CAD build for the part. Positions are in the model's coordinates, mm. A direction names the side the tool comes from. Give positions to 0.01 mm unless a question says otherwise; leave off trailing zeros. Write each loop counter-clockwise with the first axis right and the second up, starting at its lowest first coordinate (ties: lowest second). Pieces come first, ordered by that corner, then holes. Notation, with made-up numbers: (21, -4) -> (28, -4) arc R18 cw to (28, 27) -> close; hole circle Ø11 at (24.25, -34.5). An arc over 180 degrees is marked (long way). Answer in a Markdown table with one row per item. Add a question column.
```python
from build123d import *

# Parameters (mm, degrees)
SKETCH1_W           = 115
SKETCH1_H           = 70
BOSS_EXTRUDE1_DEPTH = 10
SKETCH2_R           = 6.3
SKETCH2_R_2         = 1.5
CUT_EXTRUDE1_DEPTH  = 10
SKETCH3_R           = 18.5
CUT_EXTRUDE2_DEPTH  = 5
SKETCH4_R           = 2
CUT_EXTRUDE3_DEPTH  = 10
CUT_EXTRUDE4_START  = -10
SKETCH5_R           = 2
CUT_EXTRUDE4_DEPTH  = 10
SKETCH6_R           = 2
CUT_EXTRUDE5_DEPTH  = 5
SKETCH7_R           = 2
CUT_EXTRUDE6_DEPTH  = 10


with BuildPart() as part:
    # Sketch1 → Boss-Extrude1 (new body)
    with BuildSketch(Plane(origin=(0, 0, 0), x_dir=(1, 0, 0), z_dir=(0, 1, 0))):
        Rectangle(SKETCH1_W, SKETCH1_H)
    extrude(amount=BOSS_EXTRUDE1_DEPTH)

    # Sketch2 → Cut-Extrude1 (cut)
    with BuildSketch(Plane(origin=(0, 10, 0), x_dir=(1, 0, 0), z_dir=(0, 1, 0))):
        with Locations(Location((0, -22.5, 0), (0, 0, 270))):
            Circle(SKETCH2_R)
        with Locations(Location((15.5, -15.5, 0), (0, 0, 270))):
            Circle(SKETCH2_R_2)
        with Locations(Location((7.75, -28.923393759, 0), (0, 0, 270))):
            Circle(SKETCH2_R_2)
        with Locations(Location((-7.75, -28.923393759, 0), (0, 0, 270))):
            Circle(SKETCH2_R_2)
        with Locations(Location((-15.5, -15.5, 0), (0, 0, 270))):
            Circle(SKETCH2_R_2)
        with Locations(Location((-7.75, -2.076606241, 0), (0, 0, 270))):
            Circle(SKETCH2_R_2)
        with Locations(Location((7.75, -2.076606241, 0), (0, 0, 270))):
            Circle(SKETCH2_R_2)
    extrude(amount=-CUT_EXTRUDE1_DEPTH, mode=Mode.SUBTRACT)

    # Sketch3 → Cut-Extrude2 (cut)
    with BuildSketch(Plane.XZ):
        with Locations(Location((0, 15.5, 0), (0, 0, 270))):
            Circle(SKETCH3_R)
    extrude(amount=-CUT_EXTRUDE2_DEPTH, mode=Mode.SUBTRACT)

    # Sketch4 → Cut-Extrude3 (cut)
    with BuildSketch(Plane.ZY.offset(57.5)):
        with Locations((30, 5)):
            Circle(SKETCH4_R)
        with Locations((15, 5)):
            Circle(SKETCH4_R)
        with Locations((-5, 5)):
            Circle(SKETCH4_R)
        with Locations((-25, 5)):
            Circle(SKETCH4_R)
    extrude(amount=-CUT_EXTRUDE3_DEPTH, mode=Mode.SUBTRACT)

    # Sketch5 → Cut-Extrude4 (cut)
    with BuildSketch(Plane(origin=(57.5, 0, 0), x_dir=(0, 0, -1), z_dir=(1, 0, 0)).offset(CUT_EXTRUDE4_START)):
        with Locations(Location((-30, 5, 0), (0, 0, 180))):
            Circle(SKETCH5_R)
        with Locations(Location((-15, 5, 0), (0, 0, 180))):
            Circle(SKETCH5_R)
        with Locations(Location((5, 5, 0), (0, 0, 180))):
            Circle(SKETCH5_R)
        with Locations(Location((25, 5, 0), (0, 0, 180))):
            Circle(SKETCH5_R)
    extrude(amount=CUT_EXTRUDE4_DEPTH, mode=Mode.SUBTRACT)

    # Sketch6 → Cut-Extrude5 (cut)
    with BuildSketch(Plane(origin=(0, 0, -35), x_dir=(-1, 0, 0), z_dir=(0, 0, -1))):
        with Locations((-52.5, 5)):
            Circle(SKETCH6_R)
        with Locations((52.5, 5)):
            Circle(SKETCH6_R)
    extrude(amount=-CUT_EXTRUDE5_DEPTH, mode=Mode.SUBTRACT)

    # Sketch7 → Cut-Extrude6 (cut)
    with BuildSketch(Plane.XZ):
        with Locations(Location((42.5, 20, 0), (0, 0, 270))):
            Circle(SKETCH7_R)
        with Locations(Location((42.5, 0, 0), (0, 0, 270))):
            Circle(SKETCH7_R)
        with Locations(Location((42.5, -20, 0), (0, 0, 270))):
            Circle(SKETCH7_R)
        with Locations(Location((-42.5, -20, 0), (0, 0, 270))):
            Circle(SKETCH7_R)
        with Locations(Location((-42.5, 0, 0), (0, 0, 270))):
            Circle(SKETCH7_R)
        with Locations(Location((-42.5, 20, 0), (0, 0, 270))):
            Circle(SKETCH7_R)
        with Locations(Location((0, -20, 0), (0, 0, 270))):
            Circle(SKETCH7_R)
    extrude(amount=-CUT_EXTRUDE6_DEPTH, mode=Mode.SUBTRACT)


solid = part.part
```
Item 1: Mould opens along Z. For faces 6 (the face through (-44.452, 4.93, 20.434)), 7 (the face through (-1, 5, -35)), 8 (the face through (57.5, 5, 0)) say: released by +Z, released by -Z, zero draft, split by the parting line, or undercut.
Item 2: Drop flat-ended pins along their axis: pin 1 Ø1.2 at (x, y) = (-52.5, 5) entering from -Z; pin 2 Ø3 at (x, z) = (-42.5, 20) entering from +Y; pin 3 Ø2.5 at (y, z) = (5, 15) entering from -X; pin 4 Ø3 at (y, z) = (5, 30) entering from +X. Give the stop position or say it passes through.
Item 3: Which spindle directions (+Z, -Z, +X, -X, +Y, -Y) get a long thin tool onto all of the face, cutting with end or side? Do faces 1 (the face through (-47.5, 5, -5)), 2 (the face through (54.498, 5.088, -32.535)), 3 (the face through (47.5, 5, -5)), 4 (the face through (-11.26, 2.46, 30.18)), 5 (the face through (-1, 5, 35)). Say none if no direction does.
Item 4: Slice it at B-B, the plane z = -5. List the corners of the cut face in (x, y).
Item 5: Probe L1, parallel to X at y = 8.8, z = 15.5; L2, parallel to X at y = 7.75, z = -21; L3, parallel to X at y = 7.75, z = 2.5. List the from-to ranges inside material, lowest first. Write a range as from..to.
Item 6: Slice it at A-A, the plane x = -7.75. List the corners of the cut face in (y, z), then the cut area to 3 significant figures.
Item 7: Slice it at D-D, the plane z = 5. List the corners of the cut face in (x, y), then the cut area to 3 significant figures.
Item 8: Slice it at C-C, the plane z = 26. List the corners of the cut face in (x, y), then the cut area to 3 significant figures.
Answer key:
| question | item | result |
|---|---|---|
| 1 | face 6 | undercut |
| 1 | face 7 | released by -Z |
| 1 | face 8 | zero draft |
| 2 | pin 1 | stops at z = -30 |
| 2 | pin 2 | passes through |
| 2 | pin 3 | stops at x = -47.5 |
| 2 | pin 4 | stops at x = 47.5 |
| 3 | face 1 | -X |
| 3 | face 2 | -Z |
| 3 | face 3 | +X |
| 3 | face 4 | -Y |
| 3 | face 5 | +Z, +X, -X, +Y, -Y |
| 4 | outline | (-57.5, 0) -> (57.5, 0) -> (57.5, 3) -> (47.5, 3) -> (47.5, 7) -> (57.5, 7) -> (57.5, 10) -> (-57.5, 10) -> (-57.5, 7) -> (-47.5, 7) -> (-47.5, 3) -> (-57.5, 3) -> close |
| 5 | L1 | x = -57.5..-17, -14..14, 17..57.5 |
| 5 | L2 | x = -57.5..-44.23, -40.77..-1.73, 1.73..40.77, 44.23..57.5 |
| 5 | L3 | x = -57.5..-9.19, -6.31..6.31, 9.19..57.5 |
| 6 | outline | (0, -35) -> (10, -35) -> (10, 0.58) -> (5, 0.58) -> (5, -1.3) -> (0, -1.3) -> close; (0, 32.3) -> (5, 32.3) -> (5, 30.42) -> (10, 30.42) -> (10, 35) -> (0, 35) -> close; (5, 3.58) -> (10, 3.58) -> (10, 27.42) -> (5, 27.42) -> close |
| 6 | area | 502 mm² |
| 7 | outline | (-57.5, 0) -> (-15.23, 0) -> (-15.23, 5) -> (15.23, 5) -> (15.23, 0) -> (57.5, 0) -> (57.5, 10) -> (-57.5, 10) -> close |
| 7 | area | 998 mm² |
| 8 | outline | (-57.5, 0) -> (-15.23, 0) -> (-15.23, 5) -> (-5.24, 5) -> (-5.24, 10) -> (-57.5, 10) -> close; (5.24, 5) -> (15.23, 5) -> (15.23, 0) -> (57.5, 0) -> (57.5, 10) -> (5.24, 10) -> close |
| 8 | area | 945 mm² |
